Source: CAD feature listing. Evaluate the final solid. Frame: model axes, mm. Face numbers are marked on the shaded views. A direction names the side the tool comes from. Give positions to 0.01 mm unless a question says otherwise; leave off trailing zeros. Order: outer loops, then holes, each group sorted by start corner. A loop starts at its lowest first (then second) coordinate and runs counter-clockwise, first axis right, second up.
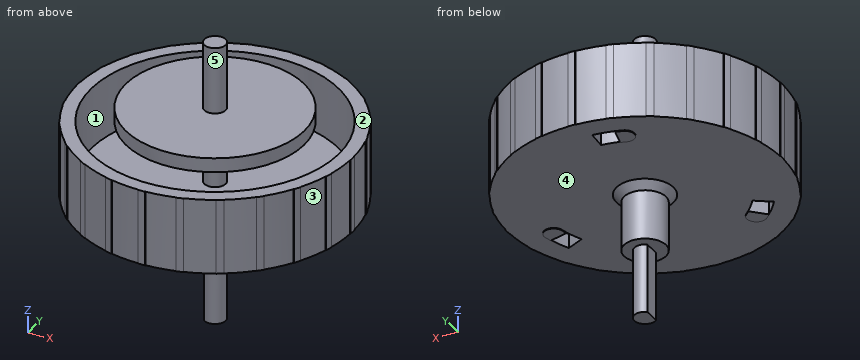
from build123d import *

# Parameters (mm, degrees)
SKETCH1_R           = 19.3
BOSS_EXTRUDE1_DEPTH = 10.6
BOSS_EXTRUDE3_DEPTH = 10.6
SKETCH8_R           = 17.35
CUT_EXTRUDE2_DEPTH  = 8.6
CIRPATTERN1_COUNT   = 24
BOSS_EXTRUDE4_DEPTH = 9.7
CUT_EXTRUDE1_DEPTH  = 11.6
BOSS_EXTRUDE5_DEPTH = 0.1
CIRPATTERN2_COUNT   = 3
SKETCH10_R          = 1.5
BOSS_EXTRUDE6_DEPTH = 20
SKETCH11_R          = 12.5
BOSS_EXTRUDE7_DEPTH = 2


with BuildPart() as part:
    # Sketch1 → Boss-Extrude1 (new body)
    with BuildSketch(Plane.XY):
        Circle(SKETCH1_R)
    extrude(amount=BOSS_EXTRUDE1_DEPTH)

    # Sketch3 → Boss-Extrude3 (add, through all)
    with BuildSketch(Plane.XY.offset(10.6)):
        with BuildLine():
            Line((-0.5, 19.343538973), (-0.49870801, 19.293555668))
            ThreePointArc((-0.49870801, 19.293555668), (0, 19.3), (0.49870801, 19.293555668))
            Line((0.49870801, 19.293555668), (0.5, 19.343538973))
            ThreePointArc((0.5, 19.343538973), (0, 19.35), (-0.5, 19.343538973))
        make_face()
    boss_extrude3 = extrude(amount=-BOSS_EXTRUDE3_DEPTH)

    # Sketch8 → Cut-Extrude2 (cut)
    with BuildSketch(Plane.XY.offset(10.6)):
        Circle(SKETCH8_R)
    extrude(amount=-CUT_EXTRUDE2_DEPTH, mode=Mode.SUBTRACT)

    # CirPattern1: Boss-Extrude3 ×24 about axis
    cirpattern1_axis = Axis((0, 0, 0), (0, 0, 1))
    for i in range(1, CIRPATTERN1_COUNT):
        add(boss_extrude3.rotate(cirpattern1_axis, i * 360 / CIRPATTERN1_COUNT))

    # Sketch5 → Revolve1 (revolve)
    with BuildSketch(Plane(origin=(0, 0, 0), x_dir=(1, 0, 0), z_dir=(0, 1, 0))):
        Polygon((0, 0), (4, 0), (2.95, 1.05), (2.95, 8), (0, 8), align=None)
    revolve(axis=Axis((0, 0, -8), (0, 0, 1)))

    # Sketch6 → Boss-Extrude4 (add)
    with BuildSketch(Plane(origin=(0, 0, -8), x_dir=(-1, 0, 0), z_dir=(0, 0, -1))):
        with BuildLine():
            Line((0.95, 1.160818677), (0.95, -1.160818677))
            ThreePointArc((0.95, -1.160818677), (-1.5, 0), (0.95, 1.160818677))
        make_face()
    extrude(amount=BOSS_EXTRUDE4_DEPTH)

    # Sketch7 → Cut-Extrude1 (cut, through all)
    with BuildSketch(Plane(origin=(0, 0, 0), x_dir=(-1, 0, 0), z_dir=(0, 0, -1))):
        with BuildLine():
            Line((1.14141791, 16.059488322), (0.95, 13.366282206))
            ThreePointArc((0.95, 13.366282206), (2.191173704, 13.219635313), (3.413286083, 12.957988969))
            Line((3.413286083, 12.957988969), (4.101037757, 15.568927045))
            ThreePointArc((4.101037757, 15.568927045), (2.632678854, 15.883293174), (1.14141791, 16.059488322))
        make_face()
    cut_extrude1 = extrude(amount=-CUT_EXTRUDE1_DEPTH, mode=Mode.SUBTRACT)

    # Sketch9 → Boss-Extrude5 (add)
    with BuildSketch(Plane(origin=(0, 0, 0), x_dir=(-1, 0, 0), z_dir=(0, 0, -1))):
        with BuildLine():
            Line((4.101037757, 15.568927045), (3.413286083, 12.957988969))
            ThreePointArc((3.413286083, 12.957988969), (3.814061699, 12.845735999), (4.211157884, 12.721090727))
            ThreePointArc((4.211157884, 12.721090727), (5.917018752, 13.578434707), (5.059674771, 15.284295574))
            Line((5.059674771, 15.284295574), (4.101037757, 15.568927045))
        make_face()
    boss_extrude5 = extrude(amount=BOSS_EXTRUDE5_DEPTH)

    # CirPattern2: Cut-Extrude1, Boss-Extrude5 ×3 about axis
    cirpattern2_axis = Axis((0, 0, 0), (0, 0, 1))
    for i in range(1, CIRPATTERN2_COUNT):
        add(cut_extrude1.rotate(cirpattern2_axis, i * 360 / CIRPATTERN2_COUNT), mode=Mode.SUBTRACT)
        add(boss_extrude5.rotate(cirpattern2_axis, i * 360 / CIRPATTERN2_COUNT))

    # Sketch10 → Boss-Extrude6 (add)
    with BuildSketch(Plane.XY.offset(2)):
        Circle(SKETCH10_R)
    extrude(amount=BOSS_EXTRUDE6_DEPTH)

    # Sketch11 → Boss-Extrude7 (add)
    with BuildSketch(Plane.XY.offset(10.6)):
        Circle(SKETCH11_R)
    extrude(amount=BOSS_EXTRUDE7_DEPTH)


solid = part.part
(1) Section B-B, the plane y = 11. Return loops of the section in (x, z).
(2) Section A-A, the plane z = 10. Count the separate pieces of the cut face and the enclosed holes in it, plus the area to 3 significant figures.
(3) Draft query along X for the marked faces 1, 2 and 3. Return one class per face: +X half, -X half, draft (parallel to the pull), parting line (faces both ways), or undercut.
(4) Access query for the marked faces 4 and 5. Directions: +Z, -Z, +X, -X, +Y, -Y. A direction counts if a zero-diameter tool reaches every point of the face in a straight line with its end or side. Return the directions, or none.
(5) Section C-C, the plane y = 6.5. Return loops of the section in (x, z), plus the area to 3 significant figures.
(6) Pin query (flat end, axial travel): pin 1 Ø1 at (x, y) = (11, -6.5) entering from +Z; pin 2 Ø10 at (x, y) = (-13, 6) entering from -Z; pin 3 Ø1 at (y, z) = (-3.5, 0.5) entering from -X. Return the tip coordinate at first contact, or that it passes through.
(7) Line query: line 1 along Y through (x, z) = (0, 8); line 2 along Z through (x, y) = (8, 0); line 3 along X through (y, z) = (1, 9.5). Output: solid intervals per line, ascending.
(8) Section D-D, the plane z = -5. Return loops of the section in (x, y).
Checks:
1. outline: (-15.86, 0) - (15.86, 0) - (15.86, 10.6) - (13.42, 10.6) - (13.42, 2) - (-13.42, 2) - (-13.42, 10.6) - (-15.86, 10.6) - close; (-5.94, 10.6) - (5.94, 10.6) - (5.94, 12.6) - (-5.94, 12.6) - close
2. separate pieces: 2
2. enclosed holes: 1
2. area: 233 mm2
3. face 1: undercut
3. face 2: draft
3. face 3: +X half
4. face 4: -Z
4. face 5: +Z
5. outline: (-18.17, 0) - (18.17, 0) - (18.17, 10.6) - (16.09, 10.6) - (16.09, 2) - (-16.09, 2) - (-16.09, 10.6) - (-18.17, 10.6) - close; (-10.68, 10.6) - (10.68, 10.6) - (10.68, 12.6) - (-10.68, 12.6) - close
5. area: 151 mm2
6. pin 1: stops at z = 12.6
6. pin 2: stops at z = 0
6. pin 3: stops at x = -19.07
7. line 1: y = -19.35 to -17.35, -1.5 to 1.5, 17.35 to 19.35
7. line 2: z = 0 to 2, 10.6 to 12.6
7. line 3: x = -19.27 to -17.32, -1.12 to 1.12, 17.32 to 19.27
8. outline: circle Ø5.9 at (0, 0)
